Work out the finished part from the listing and answer in its coordinate system (mm). Give positions to 0.01 mm unless a question says otherwise; leave off trailing zeros. One line per question, with ' | ' between items.
from build123d import *

# Parameters (mm, degrees)
SKETCH_R        = 19.5
SKETCH_R_2      = 2.2225
PAD_DEPTH       = 5.08
SKETCH030_R     = 2.2225
SKETCH030_R_2   = 19.5
POCKET_DEPTH    = 19.921
SKETCH031_R     = 1.143
POCKET001_DEPTH = 25.001


with BuildPart() as part:
    # Sketch → Pad (new body)
    with BuildSketch(Plane.XY):
        with BuildLine():
            ThreePointArc((-31.12, -23.5), (-28.888154, -28.888154), (-23.5, -31.12))
            Line((23.5, -31.12), (-23.5, -31.12))
            ThreePointArc((23.5, -31.12), (28.888154, -28.888154), (31.12, -23.5))
            Line((31.12, 23.5), (31.12, -23.5))
            ThreePointArc((31.12, 23.5), (28.888154, 28.888154), (23.5, 31.12))
            Line((-23.5, 31.12), (23.5, 31.12))
            ThreePointArc((-23.5, 31.12), (-28.888154, 28.888154), (-31.12, 23.5))
            Line((-31.12, -23.5), (-31.12, 23.5))
        make_face()
        Circle(SKETCH_R, mode=Mode.SUBTRACT)
        with Locations((-23.5, 23.5)):
            Circle(SKETCH_R_2, mode=Mode.SUBTRACT)
        with Locations((23.5, 23.5)):
            Circle(SKETCH_R_2, mode=Mode.SUBTRACT)
        with Locations((23.5, -23.5)):
            Circle(SKETCH_R_2, mode=Mode.SUBTRACT)
        with Locations((-23.5, -23.5)):
            Circle(SKETCH_R_2, mode=Mode.SUBTRACT)
    extrude(amount=PAD_DEPTH)

    # Sketch029 (on Face15 of Pad) → AdditiveLoft section 0
    with BuildSketch(Plane.XY.offset(5.08)):
        with BuildLine():
            ThreePointArc((-31.12, -23.5), (-28.888154, -28.888154), (-23.5, -31.12))
            Line((23.5, -31.12), (-23.5, -31.12))
            ThreePointArc((23.5, -31.12), (28.888154, -28.888154), (31.12, -23.5))
            Line((31.12, 23.5), (31.12, -23.5))
            ThreePointArc((31.12, 23.5), (28.888154, 28.888154), (23.5, 31.12))
            Line((-23.5, 31.12), (23.5, 31.12))
            ThreePointArc((-23.5, 31.12), (-28.888154, 28.888154), (-31.12, 23.5))
            Line((-31.12, -23.5), (-31.12, 23.5))
        make_face()
    # Sketch028 (on DatumPlane) → AdditiveLoft section 1
    with BuildSketch(Plane(origin=(0, 0, 25), x_dir=(1, 0, 0), z_dir=(0, 0, -1))):
        with BuildLine():
            ThreePointArc((-14.267762, 10.42365), (-17.145, 0), (-14.267762, -10.42365))
            Line((-14.267762, -10.42365), (-5.450863, -25.177701))
            ThreePointArc((-5.450863, -25.177701), (0, -28.27031), (5.450863, -25.177701))
            Line((5.450863, -25.177701), (14.267762, -10.42365))
            ThreePointArc((14.267762, -10.42365), (17.145, 0), (14.267762, 10.42365))
            Line((14.267762, 10.42365), (5.450863, 25.177701))
            ThreePointArc((5.450863, 25.177701), (0, 28.27031), (-5.450863, 25.177701))
            Line((-5.450863, 25.177701), (-14.267762, 10.42365))
        make_face()
    loft()

    # Sketch030 (on Face24 of AdditiveLoft) → Pocket (cut, through all)
    with BuildSketch(Plane(origin=(0, 0, 5.08), x_dir=(1, 0, 0), z_dir=(0, 0, -1))):
        with Locations((23.5, 23.5)):
            Circle(SKETCH030_R)
        Circle(SKETCH030_R_2)
        with Locations((-23.5, 23.5)):
            Circle(SKETCH030_R)
        with Locations((-23.5, -23.5)):
            Circle(SKETCH030_R)
        with Locations((23.5, -23.5)):
            Circle(SKETCH030_R)
    extrude(amount=-POCKET_DEPTH, mode=Mode.SUBTRACT)

    # Sketch031 (on Face19 of Pocket) → Pocket001 (cut, through all)
    with BuildSketch(Plane.XY.offset(25)):
        with Locations((0, 21.9202)):
            Circle(SKETCH031_R)
        with Locations((0, -21.9202)):
            Circle(SKETCH031_R)
    extrude(amount=-POCKET001_DEPTH, mode=Mode.SUBTRACT)


solid = part.part
1. Find section A-A on x = 0. State how many separate pieces and enclosed holes the cut face has, then the cut area to 3 significant figures.
Evaluation:
separate pieces: 4 | enclosed holes: 0 | area: 410 mm2
2. Consider L1, parallel to Y at x = 23.5, z = 3.25; L2, parallel to Y at x = 23.5, z = 6.5. Determine where each line is inside the solid, lowest interval first.
Evaluation:
L1: -31.12 to -25.72, -21.28 to 21.28, 25.72 to 31.12 | L2: -30.48 to -25.72, -21.28 to 21.28, 25.72 to 30.48
3. Flat-ended cylindrical pins translate along their axes: pin 1 (3 mm diameter, centred on x = 0, y = -21.92, fed in from +Z); pin 2 (5 mm diameter, centred on x = -14, z = 14.5, fed in from -Y); pin 3 (4 mm diameter, centred on x = 23.5, y = -23.5, fed in from +Z); pin 4 (5 mm diameter, centred on x = 0, z = 8, fed in from +Y). Find the tip coordinate at first contact, or state that the pin passes through.
Evaluation:
pin 1: z = 25 | pin 2: y = -29.45 | pin 3: through | pin 4: y = 31.06
4. Determine the mould class of faces 1 (the cylindrical face through (-0.842, 22.693, 12.675)), 2 (the flat face through (0, -24, 25)), 3 (the flat face through (31.12, 0, 3)) for opening direction X: +X half, -X half, draft (parallel to the pull), parting line (faces both ways), or undercut.
Evaluation:
face 1: undercut | face 2: draft | face 3: +X half
